from build123d import *

# Parameters (mm, degrees)
SKETCH_1_W             = 26
SKETCH_1_H             = 60
EXTRUDE_1_DEPTH        = 6
SKETCH_2_R             = 2
CUT_EXTRUDE_1_DEPTH    = 6
HOLE_WIZARD_M3_1_D     = 2.5
HOLE_WIZARD_M3_1_DEPTH = 7.5
HOLE_WIZARD_M3_1_TIP   = 0.751075774
CHAMFER_1_SIZE         = 5
HOLE_WIZARD_M3_2_D     = 2.5
HOLE_WIZARD_M3_2_DEPTH = 7.5
HOLE_WIZARD_M3_2_TIP   = 0.751075774


with BuildPart() as part:
    # 草图1 → 凸台-拉伸1 (new body)
    with BuildSketch(Plane.XY):
        Rectangle(SKETCH_1_W, SKETCH_1_H)
    extrude(amount=EXTRUDE_1_DEPTH)

    # 草图2 → 切除-拉伸1 (cut)
    with BuildSketch(Plane(origin=(0, 0, 0), x_dir=(-1, 0, 0), z_dir=(0, 0, -1))):
        with Locations((8, -25)):
            Circle(SKETCH_2_R)
        with Locations((-7, -25)):
            Circle(SKETCH_2_R)
        with Locations((8, 25)):
            Circle(SKETCH_2_R)
        with Locations((-7, 25)):
            Circle(SKETCH_2_R)
    extrude(amount=-CUT_EXTRUDE_1_DEPTH, mode=Mode.SUBTRACT)

    # M3 螺纹孔1
    with Locations(Plane(origin=(13, 0, 0), x_dir=(0, 0, -1), z_dir=(1, 0, 0))):
        with Locations((-3, 20), (-3, 0), (-3, -20)):
            Hole(HOLE_WIZARD_M3_1_D / 2, depth=HOLE_WIZARD_M3_1_DEPTH)
            with Locations((0, 0, -(HOLE_WIZARD_M3_1_DEPTH + HOLE_WIZARD_M3_1_TIP / 2))):  # 118° drill point
                Cone(0, HOLE_WIZARD_M3_1_D / 2, HOLE_WIZARD_M3_1_TIP, mode=Mode.SUBTRACT)

    # 倒角1
    chamfer_1_edges = [part.edges().sort_by_distance(p)[0] for p in [
        (-13, 30, 3),
        (-13, -30, 3),
    ]]
    chamfer(chamfer_1_edges, length=CHAMFER_1_SIZE)

    # M3 螺纹孔2
    with Locations(Plane.XY.offset(6)):
        with Locations((5, 5), (-5, -5)):
            Hole(HOLE_WIZARD_M3_2_D / 2, depth=HOLE_WIZARD_M3_2_DEPTH)
            with Locations((0, 0, -(HOLE_WIZARD_M3_2_DEPTH + HOLE_WIZARD_M3_2_TIP / 2))):  # 118° drill point
                Cone(0, HOLE_WIZARD_M3_2_D / 2, HOLE_WIZARD_M3_2_TIP, mode=Mode.SUBTRACT)


solid = part.part
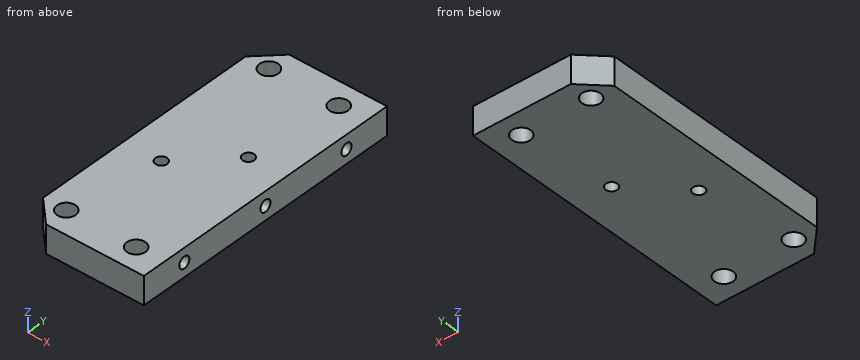
Here's how the part is built. I have some questions about the finished solid (model axes, mm). Round coordinates to 2 decimals unless told otherwise and drop trailing zeros. Loops run counter-clockwise (first coordinate to the right, second up) from the corner with the lowest first, then second, coordinate; pieces in that order, holes last. Notation, with made-up numbers: M 60,47.5 L 96,47.5 A18 ccw 96,63.5 Z; hole C 38.5,-2.5 d1. An arc over 180 degrees is marked long. Write each question's results on one line, items separated by ' | '. Start each with the question number.
(1) I want a section at B-B (z = 4.85). Please give me the cut outline in (x, y).
(2) I want a section at C-C (x = 8). Please give me the cut outline in (y, z), then the cut area to 3 significant figures.
(3) Will these pins go through, and if not, where does the flat tip stop? P1, Ø1.5, axis at x = 5, y = 5, coming from the +Z side; P2, Ø2, axis at y = 20, z = 3, coming from the +X side.
(4) I want a section at D-D (y = 5). Please give me the cut outline in (x, z).
(5) I want a section at A-A (x = -5). Please give me the cut outline in (y, z).
(6) If I drill on probe 1 along Y at (x, z) = (7, 3); probe 2 along Y at (x, z) = (10.5, 3); probe 3 along Y at (x, z) = (7.25, 5.85), over which ranges is the centre line in solid material (lowest first)? Write a range as from..to.
Solved:
1) outline: M -13,-25 L -8,-30 L 13,-30 L 13,30 L -8,30 L -13,25 Z; hole C -8,-25 d4; hole C -8,25 d4; hole C -5,-5 d2.5; hole C 5,5 d2.5; hole C 7,-25 d4; hole C 7,25 d4
2) outline: M -30,0 L -26.73,0 L -26.73,6 L -30,6 Z; M -23.27,0 L 23.27,0 L 23.27,6 L -23.27,6 Z; M 26.73,0 L 30,0 L 30,6 L 26.73,6 Z; hole C -20,3 d2.5; hole C 0,3 d2.5; hole C 20,3 d2.5 | area: 304 mm²
3) P1: passes through | P2: stops at x = 5.35
4) outline: M -13,0 L 3.75,0 L 3.75,6 L -13,6 Z; M 6.25,0 L 13,0 L 13,6 L 6.25,6 Z
5) outline: M -30,0 L -6.25,0 L -6.25,6 L -30,6 Z; M -3.75,0 L 30,0 L 30,6 L -3.75,6 Z
6) probe 1: y = -30..-27, -23..-21.25, -18.75..-1.25, 1.25..18.75, 21.25..23, 27..30 | probe 2: y = -30..-21.25, -18.75..-1.25, 1.25..18.75, 21.25..30 | probe 3: y = -30..-26.98, -23.02..23.02, 26.98..30
